Part model, mm, in its own coordinate system. A direction names the side the tool comes from. Coordinates: 2 decimals unless noted, no trailing zeros. Write each loop counter-clockwise with the first axis right and the second up, starting at its lowest first coordinate (ties: lowest second). Pieces come first, ordered by that corner, then holes. Notation, with made-up numbers: (-16.5, -9) -> (7.5, -9) arc R7 ccw to (7.5, -5) -> close; hole circle Ø1 at (21.5, -1). An arc over 180 degrees is marked (long way). One line per question, with ' | ' between items. Start each with the question number.
Item 1: 3-axis set-ups, long thin cutter, end or side, ignore diameter. For faces 1 (the flat face through (49, 10, 1)), 2 (the flat face through (20, 62, 3)): which of +Z, -Z, +X, -X, +Y, -Y reach the whole face in a straight line?
Item 2: Pin check, flat tips, straight feed: pin 1 (10 mm diameter, centred on x = 37, y = 37.5, fed in from +Z); pin 2 (0.9 mm diameter, centred on x = 49, z = 1, fed in from +Y). Stop position of each tip, or through.
Item 3: Two-plate mould, pull along Y, no slides. Class faces 3 (the flat face through (0, 129, 1)), 4 (the flat face through (4, 145, 1)), 5 (the cylindrical face through (47.5, 4.07, 1.48)), 6 (the flat face through (12.18, 58.98, 1.48)): pulls with the +Y half, pulls with the -Y half, needs draft (parallel to the pull), parting line crosses it, or undercut.
Item 4: Saw through at B-B (x = 4). List the corners of the cut face in (y, z).
Item 5: Saw through at A-A (x = 49). List the corners of the cut face in (y, z).
Item 6: Saw through at C-C (z = 1.75). List the corners of the cut face in (x, y), and give its area (3 significant figures).
Item 7: Saw through at D-D (y = 138). List the corners of the cut face in (x, z), and give its area (3 significant figures).
Item 8: Probe probe 1 along X at (y, z) = (118, 2.15); probe 2 along Y at (x, z) = (49, 0.95); probe 3 along Y at (x, z) = (48, 1.1). List the from-to ranges inside material, lowest first. Write a range as [from, to].
from build123d import *

# Parameters (mm, degrees)
SKETCH_1_R      = 1.5
EXTRUDE_1_DEPTH = 3
CHAMFER_1_SIZE  = 10
CHAMFER_1_SIZE2 = 13.076224773
FILLET_1_R      = 2


with BuildPart() as part:
    # 草图1 → 凸台-拉伸1 (new body)
    with BuildSketch(Plane.XY):
        Polygon((0, 145), (0, 115), (25, 0), (53, 0), (53, 10), (37.347826087, 10), (8, 145), align=None)
        with Locations((4, 118)):
            Circle(SKETCH_1_R, mode=Mode.SUBTRACT)
        with Locations((4, 138)):
            Circle(SKETCH_1_R, mode=Mode.SUBTRACT)
        with Locations((49, 4)):
            Circle(SKETCH_1_R, mode=Mode.SUBTRACT)
        with Locations((29, 4)):
            Circle(SKETCH_1_R, mode=Mode.SUBTRACT)
    extrude(amount=EXTRUDE_1_DEPTH)

    # 倒角1
    chamfer_1_edges = [part.edges().sort_by_distance(p)[0] for p in [
        (37.347826087, 10, 1.5),
    ]]
    chamfer_1_side = [part.faces().sort_by_distance(p)[0] for p in [
        (45.173913043, 10, 1.5),
    ]]
    chamfer(chamfer_1_edges, length=CHAMFER_1_SIZE, length2=CHAMFER_1_SIZE2, reference=chamfer_1_side[0])

    # 圆角1
    fillet_1_edges = [part.edges().sort_by_distance(p)[0] for p in [
        (8, 145, 1.5),
        (53, 10, 1.5),
        (53, 0, 1.5),
        (25, 0, 1.5),
        (0, 115, 1.5),
        (0, 145, 1.5),
    ]]
    fillet(fillet_1_edges, radius=FILLET_1_R)


solid = part.part
From the geometry:
1) face 1: +Z, -Z, +X, +Y | face 2: +Z, +X, -X, +Y, -Y
2) pin 1: through | pin 2: y = 10
3) face 3: needs draft | face 4: pulls with the +Y half | face 5: undercut | face 6: pulls with the -Y half
4) outline: (96.6, 0) -> (116.5, 0) -> (116.5, 3) -> (96.6, 3) -> close; (119.5, 0) -> (136.5, 0) -> (136.5, 3) -> (119.5, 3) -> close; (139.5, 0) -> (145, 0) -> (145, 3) -> (139.5, 3) -> close
5) outline: (0, 0) -> (2.5, 0) -> (2.5, 3) -> (0, 3) -> close; (5.5, 0) -> (10, 0) -> (10, 3) -> (5.5, 3) -> close
6) outline: (0, 115.21) arc R2 ccw to (0.05, 114.79) -> (24.66, 1.58) arc R2 ccw to (26.61, 0) -> (51, 0) arc R2 ccw to (53, 2) -> (53, 8) arc R2 ccw to (51, 10) -> (47.35, 10) -> (34.57, 22.78) -> (8.34, 143.42) arc R2 ccw to (6.39, 145) -> (2, 145) arc R2 ccw to (0, 143) -> close; hole circle Ø3 at (4, 118); hole circle Ø3 at (4, 138); hole circle Ø3 at (29, 4); hole circle Ø3 at (49, 4) | area: 2,190 mm2
7) outline: (0, 0) -> (2.5, 0) -> (2.5, 3) -> (0, 3) -> close; (5.5, 0) -> (9.52, 0) -> (9.52, 3) -> (5.5, 3) -> close | area: 19.6 mm2
8) probe 1: [0, 2.5], [5.5, 13.87] | probe 2: [0, 2.5], [5.5, 10] | probe 3: [0, 2.88], [5.12, 10]
